Print and shaded views of the part. All mm, measured from the part's lowest x, y and z. A direction names the side the tool comes from. Coordinates: 2 decimals unless noted, no trailing zeros. Loops run counter-clockwise (first coordinate to the right, second up) from the corner with the lowest first, then second, coordinate; pieces in that order, holes last. Notation, with made-up numbers: M 83.25,64.25 L 99.25,64.25 A13 ccw 99.25,79.25 Z; hole C 12.25,86 d1. An arc over 180 degrees is marked long. Use a Markdown table: item, result. Add a question column.
1) Band-saw the part on D-D (x = 15). List the corners of the cut face in (y, z), plus the area to 3 significant figures.
2) Tool access for the marked faces 1, 2 and 3: list every direction of +Z, -Z, +X, -X, +Y, -Y with a clear straight run to the whole face (end or side of a thin tool).
3) Band-saw the part on A-A (x = 2.5). List the corners of the cut face in (y, z), plus the area to 3 significant figures.
4) Wall check: probe 1 along Z at (x, y) = (15, 4.25); probe 2 along Y at (x, z) = (9.75, 34); probe 3 along Z at (x, y) = (6.5, 115). Give the ranges that are in metal, low to high. Write a range as from..to.
5) Band-saw the part on B-B (z = 15). List the corners of the cut face in (x, y), plus the area to 3 significant figures.
6) Pin check, flat tips, straight feed: pin 1 Ø3 at (x, y) = (20.5, 175) entering from -Z; pin 2 Ø16 at (x, z) = (15, 15) entering from -Y; pin 3 Ø9 at (x, z) = (16.5, 42.5) entering from -Y. Stop position of each tip, or through.
7) Band-saw the part on C-C (y = 37). List the corners of the cut face in (x, z), plus the area to 3 significant figures.
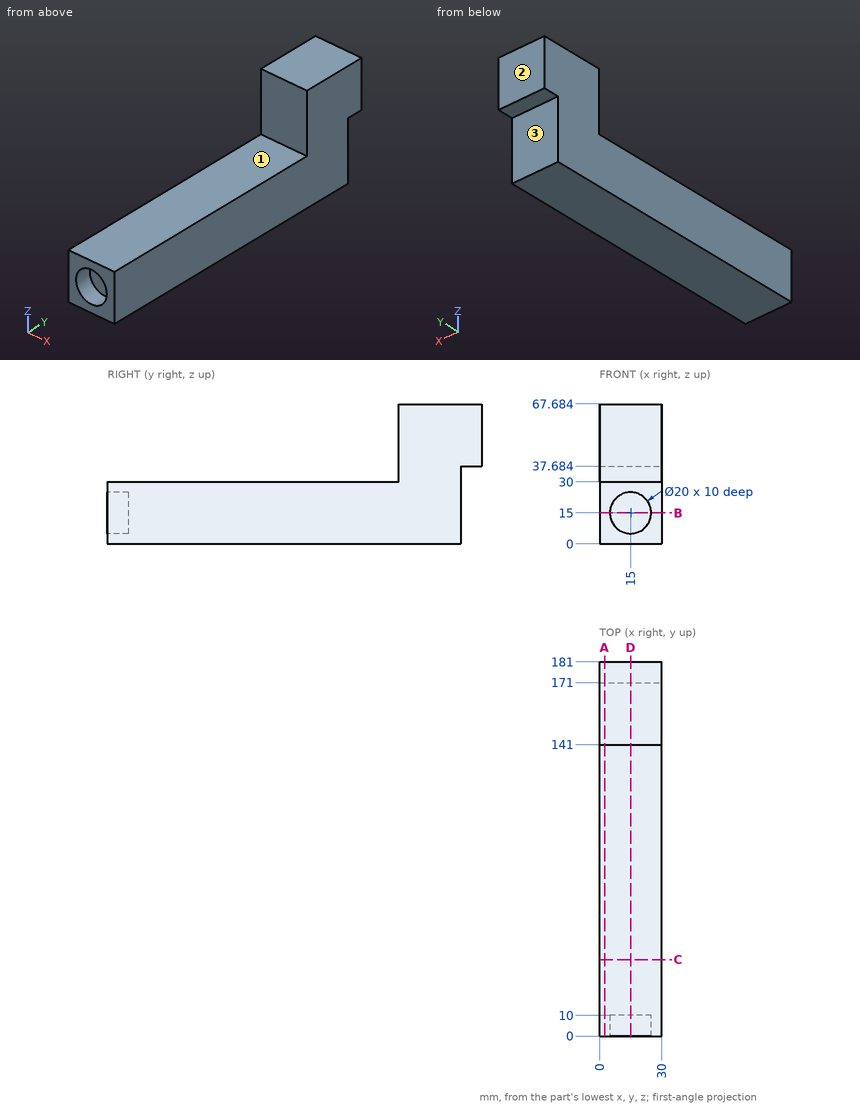
Entries:
| question | item | result |
|---|---|---|
| 1 | outline | M 0,0 L 171,0 L 171,37.68 L 181,37.68 L 181,67.68 L 141,67.68 L 141,30 L 0,30 L 0,25 L 10,25 L 10,5 L 0,5 Z |
| 1 | area | 6,360 mm2 |
| 2 | face 1 | +Z, +X, -X, -Y |
| 2 | face 2 | +Z, -Z, +X, -X, +Y |
| 2 | face 3 | -Z, +X, -X, +Y |
| 3 | outline | M 0,0 L 171,0 L 171,37.68 L 181,37.68 L 181,67.68 L 141,67.68 L 141,30 L 0,30 Z |
| 3 | area | 6,560 mm2 |
| 4 | probe 1 | 0..5, 25..30 |
| 4 | probe 2 | 141..171 |
| 4 | probe 3 | 0..30 |
| 5 | outline | M 0,0 L 5,0 L 5,10 L 25,10 L 25,0 L 30,0 L 30,171 L 0,171 Z |
| 5 | area | 4,930 mm2 |
| 6 | pin 1 | z = 37.68 |
| 6 | pin 2 | y = 10 |
| 6 | pin 3 | y = 141 |
| 7 | outline | M 0,0 L 30,0 L 30,30 L 0,30 Z |
| 7 | area | 900 mm2 |
